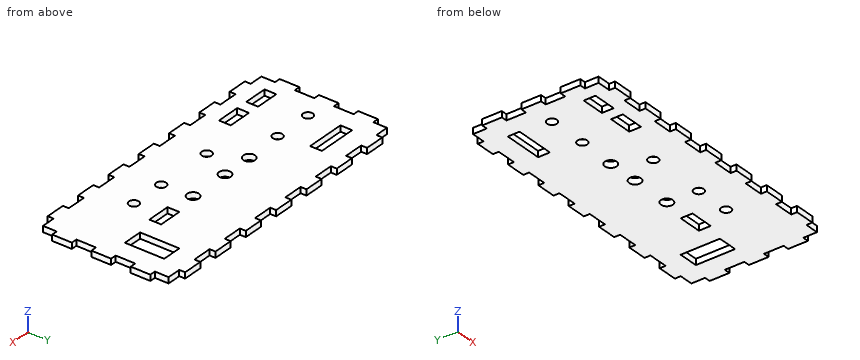
```python
from build123d import *

# Parameters (mm, degrees)
SKETCH1_W               = 150
SKETCH1_H               = 70
BOSS_EXTRUDE1_DEPTH     = 3
SKETCH2_W               = 10
SKETCH2_H               = 3
CUT_EXTRUDE1_DEPTH      = 3
LPATTERN3_COUNT         = 8
LPATTERN3_PITCH         = 20
MIRROR1_COPY_1_SKETCH_W = 10
MIRROR1_COPY_1_SKETCH_H = 3
MIRROR1_COPY_1_DEPTH    = 3
MIRROR1_COPY_2_SKETCH_W = 10
MIRROR1_COPY_2_SKETCH_H = 3
MIRROR1_COPY_2_DEPTH    = 3
MIRROR1_COPY_3_SKETCH_W = 10
MIRROR1_COPY_3_SKETCH_H = 3
MIRROR1_COPY_3_DEPTH    = 3
MIRROR1_COPY_4_SKETCH_W = 10
MIRROR1_COPY_4_SKETCH_H = 3
MIRROR1_COPY_4_DEPTH    = 3
MIRROR1_COPY_5_SKETCH_W = 10
MIRROR1_COPY_5_SKETCH_H = 3
MIRROR1_COPY_5_DEPTH    = 3
MIRROR1_COPY_6_SKETCH_W = 10
MIRROR1_COPY_6_SKETCH_H = 3
MIRROR1_COPY_6_DEPTH    = 3
MIRROR1_COPY_7_SKETCH_W = 10
MIRROR1_COPY_7_SKETCH_H = 3
MIRROR1_COPY_7_DEPTH    = 3
SKETCH3_W               = 3
SKETCH3_H               = 10
CUT_EXTRUDE2_DEPTH      = 3
LPATTERN4_COUNT         = 4
LPATTERN4_PITCH         = 20
MIRROR2_COPY_1_SKETCH_W = 3
MIRROR2_COPY_1_SKETCH_H = 10
MIRROR2_COPY_1_DEPTH    = 3
MIRROR2_COPY_2_SKETCH_W = 3
MIRROR2_COPY_2_SKETCH_H = 10
MIRROR2_COPY_2_DEPTH    = 3
MIRROR2_COPY_3_SKETCH_W = 3
MIRROR2_COPY_3_SKETCH_H = 10
MIRROR2_COPY_3_DEPTH    = 3
SKETCH4_W               = 20
SKETCH4_H               = 6
CUT_EXTRUDE3_DEPTH      = 3
SKETCH5_R               = 2.5
CUT_EXTRUDE5_DEPTH      = 3
SKETCH6_W               = 12
SKETCH6_H               = 6
CUT_EXTRUDE6_DEPTH      = 3
SKETCH7_R               = 3
CUT_EXTRUDE7_DEPTH      = 3
SKETCH8_R               = 2.5
CUT_EXTRUDE8_DEPTH      = 3
SKETCH9_R               = 3
CUT_EXTRUDE9_DEPTH      = 3
SKETCH10_W              = 12
SKETCH10_H              = 6
CUT_EXTRUDE10_DEPTH     = 3
SKETCH11_R              = 2.5
CUT_EXTRUDE11_DEPTH     = 3
SKETCH12_W              = 10
SKETCH12_H              = 20
CUT_EXTRUDE12_DEPTH     = 3


with BuildPart() as part:
    # Sketch1 → Boss-Extrude1 (new body)
    with BuildSketch(Plane.XY):
        Rectangle(SKETCH1_W, SKETCH1_H)
    extrude(amount=BOSS_EXTRUDE1_DEPTH)

    # Sketch2 → Cut-Extrude1 (cut)
    with BuildSketch(Plane.XY.offset(3)):
        with Locations((-70, 33.5)):
            Rectangle(SKETCH2_W, SKETCH2_H)
    cut_extrude1 = extrude(amount=-CUT_EXTRUDE1_DEPTH, mode=Mode.SUBTRACT)

    # LPattern3: Cut-Extrude1 ×8
    with Locations(*[(i * LPATTERN3_PITCH, 0, 0) for i in range(1, LPATTERN3_COUNT)]):
        add(cut_extrude1, mode=Mode.SUBTRACT)

    # Mirror1: Cut-Extrude1 across plane
    add(cut_extrude1.mirror(Plane.ZX), mode=Mode.SUBTRACT)

    # Mirror1 copy 1 sketch → Mirror1 copy 1 (cut)
    with BuildSketch(Plane(origin=(20, 0, 3), x_dir=(1, 0, 0), z_dir=(0, 0, 1))):
        with Locations((-70, -33.5)):
            Rectangle(MIRROR1_COPY_1_SKETCH_W, MIRROR1_COPY_1_SKETCH_H)
    extrude(amount=-MIRROR1_COPY_1_DEPTH, mode=Mode.SUBTRACT)

    # Mirror1 copy 2 sketch → Mirror1 copy 2 (cut)
    with BuildSketch(Plane(origin=(40, 0, 3), x_dir=(1, 0, 0), z_dir=(0, 0, 1))):
        with Locations((-70, -33.5)):
            Rectangle(MIRROR1_COPY_2_SKETCH_W, MIRROR1_COPY_2_SKETCH_H)
    extrude(amount=-MIRROR1_COPY_2_DEPTH, mode=Mode.SUBTRACT)

    # Mirror1 copy 3 sketch → Mirror1 copy 3 (cut)
    with BuildSketch(Plane(origin=(60, 0, 3), x_dir=(1, 0, 0), z_dir=(0, 0, 1))):
        with Locations((-70, -33.5)):
            Rectangle(MIRROR1_COPY_3_SKETCH_W, MIRROR1_COPY_3_SKETCH_H)
    extrude(amount=-MIRROR1_COPY_3_DEPTH, mode=Mode.SUBTRACT)

    # Mirror1 copy 4 sketch → Mirror1 copy 4 (cut)
    with BuildSketch(Plane(origin=(80, 0, 3), x_dir=(1, 0, 0), z_dir=(0, 0, 1))):
        with Locations((-70, -33.5)):
            Rectangle(MIRROR1_COPY_4_SKETCH_W, MIRROR1_COPY_4_SKETCH_H)
    extrude(amount=-MIRROR1_COPY_4_DEPTH, mode=Mode.SUBTRACT)

    # Mirror1 copy 5 sketch → Mirror1 copy 5 (cut)
    with BuildSketch(Plane(origin=(100, 0, 3), x_dir=(1, 0, 0), z_dir=(0, 0, 1))):
        with Locations((-70, -33.5)):
            Rectangle(MIRROR1_COPY_5_SKETCH_W, MIRROR1_COPY_5_SKETCH_H)
    extrude(amount=-MIRROR1_COPY_5_DEPTH, mode=Mode.SUBTRACT)

    # Mirror1 copy 6 sketch → Mirror1 copy 6 (cut)
    with BuildSketch(Plane(origin=(120, 0, 3), x_dir=(1, 0, 0), z_dir=(0, 0, 1))):
        with Locations((-70, -33.5)):
            Rectangle(MIRROR1_COPY_6_SKETCH_W, MIRROR1_COPY_6_SKETCH_H)
    extrude(amount=-MIRROR1_COPY_6_DEPTH, mode=Mode.SUBTRACT)

    # Mirror1 copy 7 sketch → Mirror1 copy 7 (cut)
    with BuildSketch(Plane(origin=(140, 0, 3), x_dir=(1, 0, 0), z_dir=(0, 0, 1))):
        with Locations((-70, -33.5)):
            Rectangle(MIRROR1_COPY_7_SKETCH_W, MIRROR1_COPY_7_SKETCH_H)
    extrude(amount=-MIRROR1_COPY_7_DEPTH, mode=Mode.SUBTRACT)

    # Sketch3 → Cut-Extrude2 (cut)
    with BuildSketch(Plane.XY.offset(3)):
        with Locations((-73.5, 30)):
            Rectangle(SKETCH3_W, SKETCH3_H)
    cut_extrude2 = extrude(amount=-CUT_EXTRUDE2_DEPTH, mode=Mode.SUBTRACT)

    # LPattern4: Cut-Extrude2 ×4
    with Locations(*[(0, -i * LPATTERN4_PITCH, 0) for i in range(1, LPATTERN4_COUNT)]):
        add(cut_extrude2, mode=Mode.SUBTRACT)

    # Mirror2: Cut-Extrude2 across plane
    add(cut_extrude2.mirror(Plane(origin=(0, 0, 0), x_dir=(0, 0, 1), z_dir=(1, 0, 0))), mode=Mode.SUBTRACT)

    # Mirror2 copy 1 sketch → Mirror2 copy 1 (cut)
    with BuildSketch(Plane(origin=(0, -20, 3), x_dir=(-1, 0, 0), z_dir=(0, 0, 1))):
        with Locations((-73.5, -30)):
            Rectangle(MIRROR2_COPY_1_SKETCH_W, MIRROR2_COPY_1_SKETCH_H)
    extrude(amount=-MIRROR2_COPY_1_DEPTH, mode=Mode.SUBTRACT)

    # Mirror2 copy 2 sketch → Mirror2 copy 2 (cut)
    with BuildSketch(Plane(origin=(0, -40, 3), x_dir=(-1, 0, 0), z_dir=(0, 0, 1))):
        with Locations((-73.5, -30)):
            Rectangle(MIRROR2_COPY_2_SKETCH_W, MIRROR2_COPY_2_SKETCH_H)
    extrude(amount=-MIRROR2_COPY_2_DEPTH, mode=Mode.SUBTRACT)

    # Mirror2 copy 3 sketch → Mirror2 copy 3 (cut)
    with BuildSketch(Plane(origin=(0, -60, 3), x_dir=(-1, 0, 0), z_dir=(0, 0, 1))):
        with Locations((-73.5, -30)):
            Rectangle(MIRROR2_COPY_3_SKETCH_W, MIRROR2_COPY_3_SKETCH_H)
    extrude(amount=-MIRROR2_COPY_3_DEPTH, mode=Mode.SUBTRACT)

    # Sketch4 → Cut-Extrude3 (cut)
    with BuildSketch(Plane.XY.offset(3)):
        with Locations((-52, 19)):
            Rectangle(SKETCH4_W, SKETCH4_H)
    extrude(amount=-CUT_EXTRUDE3_DEPTH, mode=Mode.SUBTRACT)

    # Sketch5 → Cut-Extrude5 (cut)
    with BuildSketch(Plane.XY.offset(3)):
        with Locations((-60, 1)):
            Circle(SKETCH5_R)
        with Locations((-40, 1)):
            Circle(SKETCH5_R)
    extrude(amount=-CUT_EXTRUDE5_DEPTH, mode=Mode.SUBTRACT)

    # Sketch6 → Cut-Extrude6 (cut)
    with BuildSketch(Plane.XY.offset(3)):
        with Locations((-59, -22)):
            Rectangle(SKETCH6_W, SKETCH6_H)
        with Locations((-41, -22)):
            Rectangle(SKETCH6_W, SKETCH6_H)
    extrude(amount=-CUT_EXTRUDE6_DEPTH, mode=Mode.SUBTRACT)

    # Sketch7 → Cut-Extrude7 (cut)
    with BuildSketch(Plane.XY.offset(3)):
        with Locations((-20, 2)):
            Circle(SKETCH7_R)
        with Locations((-4, 2)):
            Circle(SKETCH7_R)
    extrude(amount=-CUT_EXTRUDE7_DEPTH, mode=Mode.SUBTRACT)

    # Sketch8 → Cut-Extrude8 (cut)
    with BuildSketch(Plane.XY.offset(3)):
        with Locations((-12, -13.5)):
            Circle(SKETCH8_R)
    extrude(amount=-CUT_EXTRUDE8_DEPTH, mode=Mode.SUBTRACT)

    # Sketch9 → Cut-Extrude9 (cut)
    with BuildSketch(Plane.XY.offset(3)):
        with Locations((17, 2)):
            Circle(SKETCH9_R)
    extrude(amount=-CUT_EXTRUDE9_DEPTH, mode=Mode.SUBTRACT)

    # Sketch10 → Cut-Extrude10 (cut)
    with BuildSketch(Plane.XY.offset(3)):
        with Locations((36, 2)):
            Rectangle(SKETCH10_W, SKETCH10_H)
    extrude(amount=-CUT_EXTRUDE10_DEPTH, mode=Mode.SUBTRACT)

    # Sketch11 → Cut-Extrude11 (cut)
    with BuildSketch(Plane.XY.offset(3)):
        with Locations((18, -13.5)):
            Circle(SKETCH11_R)
        with Locations((36, -13.5)):
            Circle(SKETCH11_R)
    extrude(amount=-CUT_EXTRUDE11_DEPTH, mode=Mode.SUBTRACT)

    # Sketch12 → Cut-Extrude12 (cut)
    with BuildSketch(Plane.XY.offset(3)):
        with Locations((57, 12)):
            Rectangle(SKETCH12_W, SKETCH12_H)
    extrude(amount=-CUT_EXTRUDE12_DEPTH, mode=Mode.SUBTRACT)


solid = part.part
```
Geometry check sheet. Reference: the model listing, model coordinates, mm. Give positions to 0.01 mm unless a question says otherwise; leave off trailing zeros. Order: outer loops, then holes, each group sorted by start corner. A loop starts at its lowest first (then second) coordinate and runs counter-clockwise, first axis right, second up. Notation, with made-up numbers: (52, 88.5) - (89, 88.5) arc R13 cw to (89, 106.5) - close; hole circle Ø6 at (32.5, 9). An arc over 180 degrees is marked (long way). Write item = value, one per line. Start each with the question number.
1) Section check A-A (x = -20). Enter the section's corners in (y, z), then the cut area to 3 significant figures.
2) Section check B-B (y = -13.5). Enter the section's corners in (x, z), then the cut area to 3 significant figures.
3) Section check C-C (x = 18). Enter the section's corners in (y, z).
4) Gauge pin test, flat ends, axial feed: pin 1 Ø0.9 at (y, z) = (-34, 1) entering from -X; pin 2 Ø1.5 at (y, z) = (-34, 2) entering from +X; pin 3 Ø0.9 at (x, z) = (73, 1) entering from +Y. Record the tip position at first contact, or that the pin passes through.
5) Scan lines: L1, parallel to X at y = 19, z = 2.25; L2, parallel to Y at x = -40, z = 0.65; L3, parallel to Y at x = -60, z = 1.2. Record each from-to range of solid material in increasing order.
6) Section check D-D (z = 0.6). Count the separate pieces of the cut face and the enclosed holes in it, then the cut area to 3 significant figures.
Geometry check:
q1.outline = (-35, 0) - (-1, 0) - (-1, 3) - (-35, 3) - close; (5, 0) - (35, 0) - (35, 3) - (5, 3) - close
q1.area = 192 mm2
q2.outline = (-72, 0) - (-14.5, 0) - (-14.5, 3) - (-72, 3) - close; (-9.5, 0) - (15.5, 0) - (15.5, 3) - (-9.5, 3) - close; (20.5, 0) - (33.5, 0) - (33.5, 3) - (20.5, 3) - close; (38.5, 0) - (72, 0) - (72, 3) - (38.5, 3) - close
q2.area = 387 mm2
q3.outline = (-35, 0) - (-16, 0) - (-16, 3) - (-35, 3) - close; (-11, 0) - (-0.83, 0) - (-0.83, 3) - (-11, 3) - close; (4.83, 0) - (35, 0) - (35, 3) - (4.83, 3) - close
q4.pin_1 = -65
q4.pin_2 = 65
q4.pin_3 = 25
q5.L1 = -75 to -62, -42 to 52, 62 to 75
q5.L2 = -35 to -25, -19 to -1.5, 3.5 to 35
q5.L3 = -35 to -25, -19 to -1.5, 3.5 to 16, 22 to 35
q6.separate_pieces = 1
q6.enclosed_holes = 13
q6.area = 9,100 mm2
